from build123d import *

# Parameters (mm, degrees)
F1_DEPTH = 25.4
F2_DEPTH = 7.62
F3_R     = 2.54


with BuildPart() as f1:
    # F0 (on Front) → F1 (new body)
    with BuildSketch(Plane.XZ):
        with BuildLine():
            Line((0, 3.566337), (0, 10.388896))
            ThreePointArc((0, 10.388896), (-6.948698, 18.80843), (2.63599, 24.034012))
            ThreePointArc((2.63599, 24.034012), (11.508331, 28.468624), (6.047268, 36.748782))
            ThreePointArc((6.047268, 36.748782), (-11.397136, 35.333267), (-26.514942, 26.514944))
            ThreePointArc((-26.514942, 26.514944), (-41.759535, 22.502372), (-53.495057, 33.027384))
            ThreePointArc((-53.495057, 33.027384), (-62.960481, 40.999747), (-74.582964, 36.748782))
            ThreePointArc((-74.582964, 36.748782), (-82.902194, 11.322615), (-71.481802, -12.869826))
            ThreePointArc((-71.481802, -12.869826), (-57.566104, -17.244824), (-45.432035, -9.14843))
            ThreePointArc((-45.432035, -9.14843), (-32.266086, -0.852213), (-17.831687, -6.6675))
            ThreePointArc((-17.831687, -6.6675), (-5.763119, -14.325014), (8.528198, -14.11029))
            ThreePointArc((8.528198, -14.11029), (11.825983, -9.613605), (8.528198, -5.116919))
            ThreePointArc((8.528198, -5.116919), (4.464289, -3.775638), (0.438227, -2.324702))
            Line((0.438227, -2.324702), (0, 3.566337))
        make_face()
    extrude(amount=F1_DEPTH)

    # F0 (on Front) → F2 (join)
    with BuildSketch(Plane.XZ):
        Polygon((91.329239, 10.388896), (0, 10.388896), (0, 3.566337), (98.772034, 3.566337), (98.772034, 10.388896), align=None)
    extrude(amount=F2_DEPTH)

    # F3
    f3_edges = [f1.edges().sort_by_distance(p)[0] for p in [
        (49.386017, -7.62, 3.566337),
        (49.386017, -7.62, 10.388896),
    ]]
    fillet(f3_edges, radius=F3_R)


solid = f1.part
Part model, mm, in its own coordinate system. A direction names the side the tool comes from. Coordinates: 2 decimals unless noted, no trailing zeros. Write each loop counter-clockwise with the first axis right and the second up, starting at its lowest first coordinate (ties: lowest second). Pieces come first, ordered by that corner, then holes. Notation, with made-up numbers: M 40,9 L 67,9 A27 ccw 67,25 Z; hole C 67.5,72.25 d8. An arc over 180 degrees is marked long. Return JSON: item names as keys, results as strings.
1. Probe L1, parallel to Z at x = 85.5, y = -3; L2, parallel to X at y = -15.25, z = 27; L3, parallel to X at y = -13, z = -11. List the from-to ranges inside material, lowest first.
Determined:
{"L1": "3.57 to 10.39", "L2": "-80.39 to -49.7, -25.99 to 10.92", "L3": "-73.34 to -46.71, -12.93 to 11.62"}
2. 3-axis set-ups, long thin cutter, end or side, ignore diameter. For faces 1 (the face through (-5.96, -12.52, -14.27)), 2 (the face through (4.521, -12.522, -3.795)): which of +Z, -Z, +X, -X, +Y, -Y reach the whole face in a straight line?
Determined:
{"face 1": "-Z, +Y, -Y", "face 2": "+X, +Y, -Y"}
3. Saw through at B-B, the plane y = -10. Write the cut outline in (x, z), then the cut area to 3 significant figures.
Determined:
{"outline": "M -74.58,36.75 A36.19 ccw -71.48,-12.87 A16.89 ccw -45.43,-9.15 A17.09 cw -17.83,-6.67 A24.97 ccw 8.53,-14.11 A4.71 ccw 8.53,-5.12 A157.88 cw 0.44,-2.32 L 0,3.57 L 0,10.39 A7.08 cw long 2.64,24.03 A6.63 ccw long 6.05,36.75 A39.47 ccw -26.51,26.51 A16.62 cw -53.5,33.03 A12.34 ccw Z", "area": "3,560 mm²"}
4. Pull direction X, two halves, no side cores. Call faces 3 (the face through (0, -17, 7)), 4 (the face through (49, -3, 3.566)), 5 (the face through (-62.782, -12.522, 40.967)), 6 (the face through (-32.491, -12.522, -0.874)): pulls with the +X half, pulls with the -X half, needs draft (parallel to the pull), parting line crosses it, or undercut.
Determined:
{"face 3": "pulls with the +X half", "face 4": "needs draft", "face 5": "undercut", "face 6": "undercut"}
5. Saw through at A-A, the plane x = 31.5. Write the cut outline in (y, z).
Determined:
{"outline": "M -7.62,6.11 A2.54 ccw -5.08,3.57 L 0,3.57 L 0,10.39 L -5.08,10.39 A2.54 ccw -7.62,7.85 Z"}
6. Saw through at C-C, the plane z = 20. Write the cut outline in (x, y), then the cut area to 3 significant figures.
Determined:
{"outline": "M -82.4,-25.4 L -6.61,-25.4 L -6.61,0 L -82.4,0 Z", "area": "1,930 mm²"}
7. Flat gauge pins, fed straight in: pin 1 Ø1.4 at (x, z) = (53, 7) entering from -Y; pin 2 Ø3 at (x, y) = (-27, -5.5) entering from -Z; pin 3 Ø6 at (y, z) = (-7, 10.5) entering from +X; pin 4 Ø2.5 at (x, y) = (41.5, -2) entering from -Z. Where does each tip first touch, or does it go through?
Determined:
{"pin 1": "y = -7.62", "pin 2": "z = -1.61", "pin 3": "x = 98.77", "pin 4": "z = 3.57"}
